Geometry: final body of the model. Coordinates: model frame, mm. Face numbers are marked on the shaded views. A direction names the side the tool comes from. Coordinates: 2 decimals unless noted, no trailing zeros. Order: outer loops, then holes, each group sorted by start corner. A loop starts at its lowest first (then second) coordinate and runs counter-clockwise, first axis right, second up. Notation, with made-up numbers: M -6,41 L 30,41 A8 cw 30,45 Z; hole C -5,49.25 d6. An arc over 180 degrees is marked long. Use CSV: the item, a comma, the result in double quotes. Start each with the question number.
Q1. Mould query, pull axis Y, two halves, no side actions, for the marked faces 3, 4 and 5. Classes: +Y half, -Y half, draft (parallel to the pull), parting line (faces both ways), or undercut.
Q2. Section query A-A, the plane z = 41. Output: boundary loops of the cut face in (x, y), and give its area (3 significant figures).
Q3. Section query B-B, the plane z = 64.5. State how many separate pieces and enclosed holes the cut face has, and give its area (3 significant figures).
Q4. Ray query, probe 1 along Y at (x, z) = (0, 37.5); probe 2 along X at (y, z) = (-23, 43.5); probe 3 along X at (y, z) = (8, 36). Return the intervals inside material, ascending.
Q5. Access query for the marked faces 1 and 2. Directions: +Z, -Z, +X, -X, +Y, -Y. A direction counts if a zero-diameter tool reaches every point of the face in a straight line with its end or side. Return the directions, or none.
Q6. First-contact query: P1, Ø3, axis at x = -7, y = -65.5, coming from the -Z side; P2, Ø3, axis at x = -16, y = 36, coming from the +Z side; P3, Ø10, axis at x = 68, z = 37, coming from the +Y side. Flat tips, straight axial feed; report the tip coordinate or a pass-through.
Solid Edge part; units mm, degrees
sketch "Sketch1" plane through (0, 0, 0) normal (0, 0, 1) x (1, 0, 0)
  circle A0 centre (0, 0) radius 110
  circle A1 centre (0, 0) radius 70
extrude "Protrusion1" add sketch "Sketch1" along normal blind 100
fillet "Verrundung_1" radius 10 2 edges at (-110, 0, 100) (-110, 0, 0)
sketch "Sketch2" plane through (0, 0, 30) normal (0, 0, 1) x (1, 0, 0)
  circle A0 centre (0, 0) radius 25
  circle A1 centre (0, 0) radius 12.5
extrude "Extrusionsausprägung_2" add sketch "Sketch2" along normal blind 30
sketch "Sketch3" plane through (0, 0, 0) normal (0, -1, 0) x (1, 0, 0)
  line L0 (70, 100) -> (70, 90)
  spline S0 degree 3 poles (25, 50) (39.5289, 80.1519) (54.5289, 93.4852) (70, 90) knots 0 0 0 0 1 1 1 1
  line L1 (25, 60) -> (25, 50)
  spline S1 degree 3 poles (25, 60) (34.2198, 86.6371) (49.2198, 99.9704) (70, 100) knots 0 0 0 0 1 1 1 1
  dimension "D1" = 70
  dimension "D2" = 25
revolve "Rotationsausprägung_1" add sketch "Sketch3" angle 20 about axis through (0, 0, 54) along (0, 0, 1)
pattern_circular "Pattern1" count 11 over 360 about axis through (0, 0, 100) along (0, 0, 1) of "Rotationsausprägung_1"
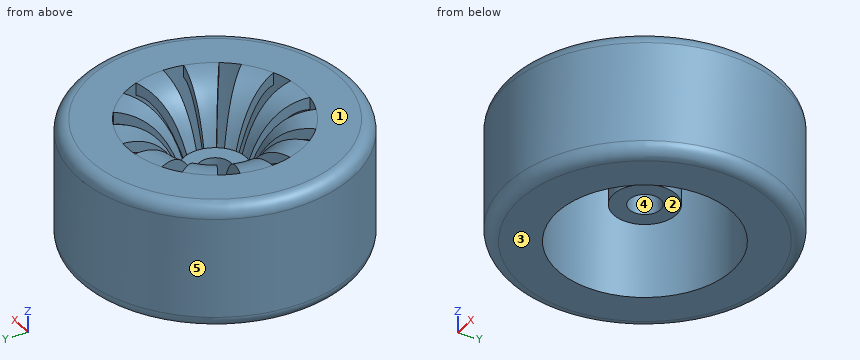
Responses:
1,face 3,"draft"
1,face 4,"undercut"
1,face 5,"parting line"
2,outline,"C 0,0 d220; C 0,0 d50; hole C 0,0 d140; hole C 0,0 d25"
2,area,"24,100 mm²"
3,separate pieces,"12"
3,enclosed holes,"1"
3,area,"23,300 mm²"
4,probe 1,"y = -110 to -70, -25 to -12.5, 12.5 to 25, 70 to 110"
4,probe 2,"x = -107.57 to -66.11, -9.8 to 9.8, 66.11 to 107.57"
4,probe 3,"x = -109.71 to -69.54, -23.69 to -9.6, 9.6 to 23.69, 69.54 to 109.71"
5,face 1,"+Z, +X, -X, +Y, -Y"
5,face 2,"-Z"
6,P1,"stops at z = 90.43"
6,P2,"stops at z = 87.81"
6,P3,"stops at y = 90.17"
